```python
from build123d import *

# Parameters (mm, degrees)
SKETCH1_W           = 12
SKETCH1_H           = 4.42
SKETCH1_W_2         = 11.36
SKETCH1_H_2         = 3.78
SKETCH1_H_3         = 1.68
BOSS_EXTRUDE1_DEPTH = 11.8
BOSS_EXTRUDE3_DEPTH = 14
SKETCH3_R           = 2.96
BOSS_EXTRUDE4_DEPTH = 5.92
CUT_EXTRUDE1_REACH  = 7.72
SKETCH4_W           = 2
SKETCH4_H           = 1.5


with BuildPart() as part:
    # Sketch1 → Boss-Extrude1 (new body)
    with BuildSketch(Plane.XY):
        Rectangle(SKETCH1_W, SKETCH1_H)
        Rectangle(SKETCH1_W_2, SKETCH1_H_2, mode=Mode.SUBTRACT)
        with Locations((0, -1.05)):
            Rectangle(SKETCH1_W_2, SKETCH1_H_3)
    extrude(amount=-BOSS_EXTRUDE1_DEPTH)

    # Sketch2 → Boss-Extrude3 (add)
    with BuildSketch(Plane(origin=(0, 0, -11.8), x_dir=(-1, 0, 0), z_dir=(0, 0, -1))):
        with BuildLine():
            ThreePointArc((-6.132053571, 3.071220572), (-6.491568803, 2.929374125), (-6.754360741, 2.64598038))
            add(Edge.make_bspline(
                [(-6.754360741, 2.64598038), (-8.283596649, 0), (-6.754360741, -2.64598038)],
                knots=[5.839065971, 5.839065971, 5.839065971, 6.727304644, 6.727304644, 6.727304644], degree=2, weights=[1, 0.902989404, 1]))
            ThreePointArc((-6.754360741, -2.64598038), (-6.491568803, -2.929374125), (-6.132053571, -3.071220572))
            add(Edge.make_bspline(
                [(-6.132053571, -3.071220572), (0, -4.011467008), (6.132053571, -3.071220572)],
                knots=[1.065418499, 1.065418499, 1.065418499, 2.076174155, 2.076174155, 2.076174155], degree=2, weights=[1, 0.874991616, 1]))
            ThreePointArc((6.132053571, -3.071220572), (6.491568803, -2.929374125), (6.754360741, -2.64598038))
            add(Edge.make_bspline(
                [(6.754360741, -2.64598038), (8.283596649, 0), (6.754360741, 2.64598038)],
                knots=[2.697473317, 2.697473317, 2.697473317, 3.58571199, 3.58571199, 3.58571199], degree=2, weights=[1, 0.902989404, 1]))
            ThreePointArc((6.754360741, 2.64598038), (6.491568803, 2.929374125), (6.132053571, 3.071220572))
            add(Edge.make_bspline(
                [(6.132053571, 3.071220572), (0, 4.011467008), (-6.132053571, 3.071220572)],
                knots=[4.207011152, 4.207011152, 4.207011152, 5.217766808, 5.217766808, 5.217766808], degree=2, weights=[1, 0.874991616, 1]))
        make_face()
    extrude(amount=BOSS_EXTRUDE3_DEPTH)

    # Sketch3 → Boss-Extrude4 (add)
    with BuildSketch(Plane(origin=(0, 0, -25.8), x_dir=(-1, 0, 0), z_dir=(0, 0, -1))):
        Circle(SKETCH3_R)
    extrude(amount=BOSS_EXTRUDE4_DEPTH)

    # Sketch4 → Cut-Extrude1 (cut, up to next)
    with BuildSketch(Plane(origin=(0, 2.21, 0), x_dir=(1, 0, 0), z_dir=(0, 1, 0)), mode=Mode.PRIVATE) as cut_extrude1_sk1:
        with Locations((3, 5.9)):
            Rectangle(SKETCH4_W, SKETCH4_H)
    cut_extrude1_tool1 = extrude(cut_extrude1_sk1.sketch, amount=-CUT_EXTRUDE1_REACH, mode=Mode.PRIVATE) & part.part
    add(cut_extrude1_tool1.solids().sort_by_distance((3, 2.21, -5.9))[0], mode=Mode.SUBTRACT)
    # Sketch4 → Cut-Extrude1 (cut, up to next)
    with BuildSketch(Plane(origin=(0, 2.21, 0), x_dir=(1, 0, 0), z_dir=(0, 1, 0)), mode=Mode.PRIVATE) as cut_extrude1_sk2:
        with Locations((-3, 5.9)):
            Rectangle(SKETCH4_W, SKETCH4_H)
    cut_extrude1_tool2 = extrude(cut_extrude1_sk2.sketch, amount=-CUT_EXTRUDE1_REACH, mode=Mode.PRIVATE) & part.part
    add(cut_extrude1_tool2.solids().sort_by_distance((-3, 2.21, -5.9))[0], mode=Mode.SUBTRACT)


solid = part.part
```
Design review of the part built by this model. Coordinates are the model's own, in mm. A direction names the side the tool comes from. Give positions to 0.01 mm unless a question says otherwise; leave off trailing zeros. Write each loop counter-clockwise with the first axis right and the second up, starting at its lowest first coordinate (ties: lowest second). Pieces come first, ordered by that corner, then holes. Notation, with made-up numbers: (52.5, 58) -> (63.5, 58) arc R8 ccw to (63.5, 71) -> close; hole circle Ø5 at (-7, 4). An arc over 180 degrees is marked (long way). Answer in a Markdown table with one row per item.
(1) Mouldability with a two-part tool opening along Y and no side actions: class faces 6 (the flat face through (0, -2.21, -6)), 7 (the flat face through (0, 1, -11.8)), 8 (the cylindrical face through (2.35, -1.8, -28.72)) as +Y half, -Y half, draft (parallel to the pull), parting line (faces both ways), or undercut.
Results:
| item | result |
|---|---|
| face 6 | -Y half |
| face 7 | undercut |
| face 8 | parting line |
(2) For faces 1 (the flat face through (5.68, 1, -6)), 2 (the flat face through (0, 2.21, -6)), 3 (the flat face through (6, 0, -6)), 4 (the flat face through (-6, 0, -6)), 5 (the flat face through (-0.1, -0.5, 0)), list the 3-axis set-ups (+Z, -Z, +X, -X, +Y, -Y) from which the entire face can be reached by the end or side of a thin tool; tool diameter is ignored.
Results:
| item | result |
|---|---|
| face 1 | +Z |
| face 2 | +Z, +X, -X, +Y |
| face 3 | +Z, +X, +Y, -Y |
| face 4 | +Z, -X, +Y, -Y |
| face 5 | +Z, +X, -X, +Y, -Y |
(3) Clearance check with flat-ended pins moving along their axes: pin 1 (1 mm diameter, centred on y = 1, z = -3.5, fed in from -X); pin 2 (1 mm diameter, centred on y = 0.5, z = -4.5, fed in from +X); pin 3 (1 mm diameter, centred on x = 1.5, y = 0.5, fed in from +Z). State where each tip first meets the part, or that it passes through.
Results:
| item | result |
|---|---|
| pin 1 | x = -6 |
| pin 2 | x = 6 |
| pin 3 | z = -11.8 |
(4) To check wall thickness, follow probe 1 along Y at (x, z) = (-0.75, -10.5); probe 2 along X at (y, z) = (1, -10); probe 3 along Z at (x, y) = (0.5, 1). State the ranges of each line that lie inside material, in increasing order.
Results:
| item | result |
|---|---|
| probe 1 | -2.21 to -0.21, 1.89 to 2.21 |
| probe 2 | -6 to -5.68, 5.68 to 6 |
| probe 3 | -31.72 to -11.8 |
(5) Consider section A-A (z = -11). State the section outline as (x, y) points, then the cut area to 3 significant figures.
Results:
| item | result |
|---|---|
| outline | (-6, -2.21) -> (6, -2.21) -> (6, 2.21) -> (-6, 2.21) -> close; hole (-5.68, -0.21) -> (5.68, -0.21) -> (5.68, 1.89) -> (-5.68, 1.89) -> close |
| area | 29.2 mm2 |
(6) Consider section B-B (z = -5.5). State the section outline as (x, y) points.
Results:
| item | result |
|---|---|
| outline | (-6, -2.21) -> (6, -2.21) -> (6, 2.21) -> (4, 2.21) -> (4, 1.89) -> (5.68, 1.89) -> (5.68, -0.21) -> (-5.68, -0.21) -> (-5.68, 1.89) -> (-4, 1.89) -> (-4, 2.21) -> (-6, 2.21) -> close; (-2, 1.89) -> (2, 1.89) -> (2, 2.21) -> (-2, 2.21) -> close |
